Read the model definition and answer for the solid it produces. Units are mm, in the model's axes. Coordinates: 2 decimals unless noted, no trailing zeros. Loops run counter-clockwise (first coordinate to the right, second up) from the corner with the lowest first, then second, coordinate; pieces in that order, holes last.
Q1. Straight lines are drawn through the part: line 1 (Y direction, x = 1.25, z = -1); line 2 (Y direction, x = 1.75, z = -0.75); line 3 (Y direction, x = 0.75, z = 3.5). For each, find the intervals that lie inside material, in ascending order.
Q2. Section A-A (x = 3) is taken. Give the vertices of the cut face in (y, z).
Q3. The mould has two halves that part along X. Classify faces 1 (the face through (4.386, -0.168, 1.604)), 2 (the face through (5, 0, 2)), 3 (the face through (0, 0, 2)): pulls with the +X half, pulls with the -X half, needs draft (parallel to the pull), parting line crosses it, or undercut.
Q4. Section D-D (z = -1.25) is taken. Give the vertices of the cut face in (x, y), then the cut area to 3 significant figures.
Q5. Section B-B (z = 4.5) is taken. Give the vertices of the cut face in (x, y).
Q6. Section C-C (y = -6.25) is taken. Give the vertices of the cut face in (x, z), then the cut area to 3 significant figures.
Q7. A flat-ended cylindrical pin translates along its axis: P1, Ø1.3, axis at y = 8.41, z = -0.97, coming from the -X side. Find the tip coordinate at first contact, or state that the pin passes through.
Autodesk Inventor part; units mm, degrees
ref_plane "YZ Plane" through (0, 0, 0) normal (1, 0, 0) x (0, 1, 0)
ref_plane "XZ Plane" through (0, 0, 0) normal (0, 1, 0) x (-1, 0, 0)
ref_plane "XY Plane" through (0, 0, 0) normal (0, 0, 1) x (1, 0, 0)
sketch "Sketch1" plane through (0, 0, 0) normal (1, 0, 0) x (0, 1, 0)
  line L0 (-9.5937, 6.5342) -> (10.4063, 6.5342)
  line L1 (10.4063, 6.5342) -> (10.4063, -3.4658)
  line L2 (10.4063, -3.4658) -> (-9.5937, -3.4658)
  line L3 (-9.5937, -3.4658) -> (-9.5937, 6.5342)
  point P0 (0, 0)
  dimension "d0" = 20
  dimension "d1" = 10
extrude "Extrusion1" add sketch "Sketch1" along normal blind 5
sketch "Sketch2" plane through (0, -9.5937, 6.5342) normal (0, 0, 1) x (1, 0, 0)
  circle A0 centre (3, 10) radius 1.5
  line L0 (5, 20) -> (5, 0)
  line L1 (0, 20) -> (5, 20)
  point P0 (0, 9.5937)
  dimension "d4" = 3
  dimension "d5" = 2
  dimension "d6" = 10
extrude "Extrusion2" cut sketch "Sketch2" against normal through all
sketch "Sketch3" plane through (5, 0, 0) normal (1, 0, 0) x (0, 0, -1)
  circle A0 centre (-4.0342, -6.5937) radius 0.8
  circle A1 centre (0.9658, -6.5937) radius 0.8
  circle A2 centre (-4.0342, 8.4063) radius 0.8
  circle A3 centre (0.9658, 8.4063) radius 0.8
  line L0 (-6.5342, 10.4063) -> (-6.5342, -9.5937)
  line L1 (3.4658, -9.5937) -> (3.4658, 10.4063)
  line L2 (-6.5342, -9.5937) -> (3.4658, -9.5937)
  point P0 (0, 0)
  dimension "d9" = 1.6
  dimension "d11" = 1.6
  dimension "d12" = 1.6
  dimension "d13" = 1.6
  dimension "d14" = 2.5
  dimension "d15" = 2.5
  dimension "d16" = 3
  dimension "d17" = 3
  dimension "d18" = 15
  dimension "d19" = 15
  dimension "d20" = 2.5
  dimension "d21" = 2.5
extrude "Extrusion3" cut sketch "Sketch3" against normal through all
properties part number "z_shaft_block"
Numbers:
1. line 1: y = -9.59 to -7.39, -5.79 to 7.61, 9.21 to 10.41
1. line 2: y = -9.59 to -7.36, -5.82 to -0.42, 1.24 to 7.64, 9.18 to 10.41
1. line 3: y = -9.59 to -7.19, -6 to 7.81, 9 to 10.41
2. outline: (-9.59, -3.47) - (-1.09, -3.47) - (-1.09, 6.53) - (-9.59, 6.53) - close; (1.91, -3.47) - (10.41, -3.47) - (10.41, 6.53) - (1.91, 6.53) - close; hole circle Ø1.6 at (-6.59, -0.97); hole circle Ø1.6 at (-6.59, 4.03); hole circle Ø1.6 at (8.41, -0.97); hole circle Ø1.6 at (8.41, 4.03)
3. face 1: undercut
3. face 2: pulls with the +X half
3. face 3: pulls with the -X half
4. outline: (0, -9.59) - (5, -9.59) - (5, -7.34) - (0, -7.34) - close; (0, -5.85) - (5, -5.85) - (5, 7.66) - (0, 7.66) - close; (0, 9.15) - (5, 9.15) - (5, 10.41) - (0, 10.41) - close; hole circle Ø3 at (3, 0.41)
4. area: 78.0 mm2
5. outline: (0, -9.59) - (5, -9.59) - (5, -7.24) - (0, -7.24) - close; (0, -5.94) - (5, -5.94) - (5, 7.76) - (0, 7.76) - close; (0, 9.06) - (5, 9.06) - (5, 10.41) - (0, 10.41) - close; hole circle Ø3 at (3, 0.41)
6. outline: (0, -3.47) - (5, -3.47) - (5, -1.69) - (0, -1.69) - close; (0, -0.24) - (5, -0.24) - (5, 3.31) - (0, 3.31) - close; (0, 4.76) - (5, 4.76) - (5, 6.53) - (0, 6.53) - close
6. area: 35.6 mm2
7. P1: passes through
